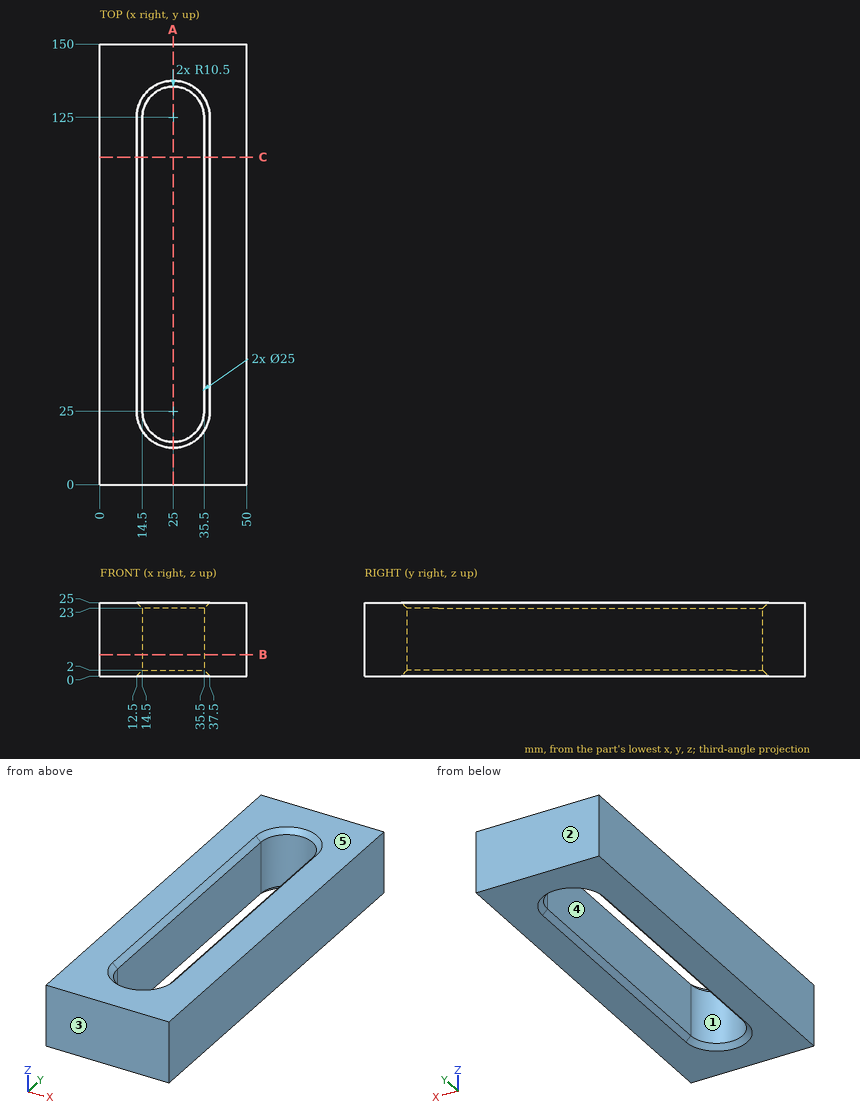
Here's the drawing with two shaded views (mm, measured from the low corner). I have some questions. A direction names the side the tool comes from. Give positions to 0.01 mm unless a question says otherwise; leave off trailing zeros. Write each loop counter-clockwise with the first axis right and the second up, starting at its lowest first coordinate (ties: lowest second). Pieces come first, ordered by that corner, then holes. Notation, with made-up numbers: (18.25, 11.25) -> (34.25, 11.25) arc R23 ccw to (34.25, 46.25) -> close; hole circle Ø6 at (59, -16.75). An arc over 180 degrees is marked (long way). Use one line per item in the form item = value.
1) We'd pull the mould along Y, two halves only. Please class the marked faces 1, 2 and 3: +Y half, -Y half, draft (parallel to the pull), parting line (faces both ways), or undercut.
Verdict:
face_1 = undercut
face_2 = +Y half
face_3 = -Y half
2) On a 3-axis mill with a long thin cutter (end or side, diameter ignored), from which of +Z, -Z, +X, -X, +Y, -Y can I reach the whole of each face in a straight line? I mean the marked faces 4 and 5. Say none if no direction works.
Verdict:
face_4 = +Z, -Z
face_5 = +Z, +X, -X, +Y, -Y
3) If I drill on L1, parallel to X at y = 113, z = 19.5; L2, parallel to Y at x = 24.5, z = 8.5; L3, parallel to Y at x = 33, z = 5.5, over which ranges is the centre line in solid material (lowest first)? Write a range as [from, to].
Verdict:
L1 = [0, 14.5], [35.5, 50]
L2 = [0, 14.51], [135.49, 150]
L3 = [0, 18.2], [131.8, 150]
4) Suppose I cut it at B-B (z = 7.25). Please give me the cut outline in (x, y).
Verdict:
outline = (0, 0) -> (50, 0) -> (50, 150) -> (0, 150) -> close; hole (14.5, 25) arc R10.5 ccw to (35.5, 25) -> (35.5, 125) arc R10.5 ccw to (14.5, 125) -> close
5) Suppose I cut it at A-A (x = 25). Please give me the cut outline in (y, z).
Verdict:
outline = (0, 0) -> (12.5, 0) -> (14.5, 2) -> (14.5, 23) -> (12.5, 25) -> (0, 25) -> close; (135.5, 2) -> (137.5, 0) -> (150, 0) -> (150, 25) -> (137.5, 25) -> (135.5, 23) -> close
6) I'm going to push a flat-ended pin straight in: pin 1 (8 mm diameter, centred on x = 18, y = 78, fed in from -Z). Where does the tip first touch, or does it pass through?
Verdict:
pin_1 = 1.5
7) Suppose I cut it at C-C (y = 111.5). Please give me the cut outline in (x, z).
Verdict:
outline = (0, 0) -> (12.5, 0) -> (14.5, 2) -> (14.5, 23) -> (12.5, 25) -> (0, 25) -> close; (35.5, 2) -> (37.5, 0) -> (50, 0) -> (50, 25) -> (37.5, 25) -> (35.5, 23) -> close
